from build123d import *

# Parameters (mm, degrees)
F0_W      = 660.4
F0_H      = 228.6
F0_W_2    = 320.675
F0_H_2    = 215.9
F1_DEPTH  = 127
F2_DEPTH  = 22.225
F3_DEPTH  = 6.35
F4_DEPTH  = 6.35
F5_DEPTH  = 6.35
F6_DEPTH  = 6.35
F7_W      = 311.15
F7_H      = 6.35
F7_W_2    = 304.7793038845
F8_DEPTH  = 31.75
F10_DEPTH = 127
F11_SIZE2 = 127
F11_SIZE  = 177.8
F12_R     = 101.6
F13_R     = 50.8


with BuildPart() as f1:
    # F0 (on Front) → F1 (new body)
    with BuildSketch(Plane.XZ):
        Rectangle(F0_W, F0_H)
        with Locations((-163.5125, 0)):
            Rectangle(F0_W_2, F0_H_2, mode=Mode.SUBTRACT)
        with Locations((163.5125, 0)):
            Rectangle(F0_W_2, F0_H_2, mode=Mode.SUBTRACT)
    extrude(amount=F1_DEPTH)

    # F2 (add, symmetric): a face of the model
    f2_faces = [f1.faces().sort_by_distance(p)[0] for p in [
        (3.175, -63.5, 0),
    ]]
    extrude(f2_faces, amount=F2_DEPTH, both=True)

    # F3 (add): a face of the model
    f3_faces = [f1.faces().sort_by_distance(p)[0] for p in [
        (330.2, -63.5, 0),
    ]]
    extrude(f3_faces, amount=F3_DEPTH)

    # F4 (cut): a face of the model
    f4_faces = [f1.faces().sort_by_distance(p)[0] for p in [
        (323.85, -63.5, 0),
    ]]
    extrude(f4_faces, amount=-F4_DEPTH, mode=Mode.SUBTRACT)

    # F5 (add): a face of the model
    f5_faces = [f1.faces().sort_by_distance(p)[0] for p in [
        (-330.2, -63.5, 0),
    ]]
    extrude(f5_faces, amount=F5_DEPTH)

    # F6 (cut): a face of the model
    f6_faces = [f1.faces().sort_by_distance(p)[0] for p in [
        (-323.85, -63.5, 0),
    ]]
    extrude(f6_faces, amount=-F6_DEPTH, mode=Mode.SUBTRACT)

    # F7 (on face) → F8 (cut)
    with BuildSketch(Plane.XZ.offset(127)):
        with Locations((-174.625, -111.125)):
            Rectangle(F7_W, F7_H)
        with Locations((177.7896519423, -111.125)):
            Rectangle(F7_W_2, F7_H)
    extrude(amount=-F8_DEPTH, mode=Mode.SUBTRACT)

    # F9 (on face) → F10 (join)
    with BuildSketch(Plane.XZ.offset(127)):
        Polygon((-19.05, 107.95), (-19.05, -114.3), (25.4, -114.3), (25.4, 107.95), (330.2, 107.95), (330.2, -107.95), (330.1793038845, -107.95), (330.1793038845, -114.3), (336.55, -114.3), (336.55, 114.3), (-336.55, 114.3), (-336.55, -114.3), (-330.2, -114.3), (-330.2, 107.95), align=None)
    extrude(amount=F10_DEPTH)

    # F11
    f11_edges = [f1.edges().sort_by_distance(p)[0] for p in [
        (3.175, -254, -114.3),
        (-333.375, -254, -114.3),
        (333.364652, -254, -114.3),
    ]]
    f11_side = f1.faces().sort_by_distance((1.850226, -254, 25.602564))[0]
    chamfer(f11_edges, length=F11_SIZE, length2=F11_SIZE2, reference=f11_side)

    # F12
    f12_edges = [f1.edges().sort_by_distance(p)[0] for p in [
        (3.175, -254, 63.5),
        (-333.375, -254, 63.5),
        (333.375, -254, 63.5),
    ]]
    fillet(f12_edges, radius=F12_R)

    # F13
    f13_edges = [f1.edges().sort_by_distance(p)[0] for p in [
        (3.175, -127, -114.3),
        (-333.375, -127, -114.3),
        (333.364652, -127, -114.3),
    ]]
    fillet(f13_edges, radius=F13_R)


solid = f1.part
Work out the finished part from the listing and answer in its coordinate system (mm). A direction names the side the tool comes from. Coordinates: 2 decimals unless noted, no trailing zeros. Write each loop counter-clockwise with the first axis right and the second up, starting at its lowest first coordinate (ties: lowest second). Pieces come first, ordered by that corner, then holes. Notation, with made-up numbers: M 5,41.25 L 56,41.25 A33 ccw 56,76.25 Z; hole C -27.5,50.25 d2. An arc over 180 degrees is marked long. Write item = value, one per line.
1. For faces 5 (the face through (-5, -50, -114.3)), 6 (the face through (-177, -125, 107.95)), determine the directions among +Z, -Z, +X, -X, +Y, -Y from which every point of the face is accessible in a straight line to the end or side of a thin tool.
Solution:
face_5 = -Z, +X, -X, +Y, -Y
face_6 = +Y, -Y
2. Determine the mould class of faces 1 (the face through (176, -125, 107.95)), 2 (the face through (-5, -254, 109)), 3 (the face through (5, -125, 114.3)), 4 (the face through (-177, -47, -107.95)) for opening direction Z: released by +Z, released by -Z, zero draft, split by the parting line, or undercut.
Solution:
face_1 = undercut
face_2 = zero draft
face_3 = released by +Z
face_4 = undercut
3. Flat-ended cylindrical pins translate along their axes: pin 1 (5 mm diameter, centred on x = -114.5, z = -112, fed in from -Y); pin 2 (1 mm diameter, centred on x = -91.5, y = -164.5, fed in from -Z). Find the tip coordinate at first contact, or state that the pin passes through.
Solution:
pin_1 = -95.25
pin_2 = 107.95
4. The part is cut by section B-B (y = -85). Determine the outline of the cut face in (x, z).
Solution:
outline = M -336.55,-114.3 L 336.55,-114.3 L 336.55,114.3 L -336.55,114.3 Z; hole M -330.2,-107.95 L -19.05,-107.95 L -19.05,107.95 L -330.2,107.95 Z; hole M 25.4,-107.95 L 330.2,-107.95 L 330.2,107.95 L 25.4,107.95 Z
5. Straight lines are drawn through the part: line 1 (X direction, y = -51, z = -87); line 2 (Z direction, x = -185, y = -45). For each, find the intervals that lie inside material, in ascending order. Write a range as from..to.
Solution:
line_1 = -336.55..-330.2, -19.05..25.4, 330.2..336.55
line_2 = -114.3..-107.95, 107.95..114.3
6. The part is cut by section C-C (z = 20.5). Determine the outline of the cut face in (x, y).
Solution:
outline = M -336.55,-223.29 L -330.2,-223.29 L -330.2,0 L -336.55,0 Z; M -19.05,-223.29 L 25.4,-223.29 L 25.4,0 L -19.05,0 Z; M 330.2,-223.29 L 336.55,-223.29 L 336.55,0 L 330.2,0 Z
7. The part is cut by section D-D (y = -202). Determine the outline of the cut face in (x, z), then the cut area to 3 significant figures.
Solution:
outline = M -336.55,-9.3 L -330.2,-9.3 L -330.2,107.95 L -19.05,107.95 L -19.05,-9.3 L 25.4,-9.3 L 25.4,107.95 L 330.2,107.95 L 330.2,-9.3 L 336.55,-9.3 L 336.55,114.3 L -336.55,114.3 Z
area = 11,000 mm2
8. The part is cut by section A-A (x = -245). Determine the outline of the cut face in (y, z).
Solution:
outline = M -254,107.95 L 0,107.95 L 0,114.3 L -254,114.3 Z; M -95.25,-114.3 L 0,-114.3 L 0,-107.95 L -95.25,-107.95 Z
